Can you work these out from the model? Positions are in its coordinate system, mm. A direction names the side the tool comes from. Round coordinates to 2 decimals unless told otherwise and drop trailing zeros. Order: outer loops, then holes, each group sorted by start corner. A loop starts at its lowest first (then second) coordinate and runs counter-clockwise, first axis right, second up. Notation, with made-up numbers: (6.5, 2) - (42.5, 2) arc R16 cw to (42.5, 27) - close; hole circle Ø1 at (39.5, -34). An arc over 180 degrees is marked (long way). Write item = value, one per line.
from build123d import *

# Parameters (mm, degrees)
SKETCH1_W           = 29
SKETCH1_H           = 35
BOSS_EXTRUDE1_DEPTH = 2
SKETCH4_W           = 3
SKETCH4_H           = 35
BOSS_EXTRUDE3_DEPTH = 2
SKETCH5_W           = 3.5
SKETCH5_H           = 1.5
SKETCH5_W_2         = 1.5
SKETCH5_H_2         = 3.7
BOSS_EXTRUDE4_DEPTH = 35
SKETCH6_W           = 2
SKETCH6_H           = 35
BOSS_EXTRUDE5_DEPTH = 35
SKETCH7_W           = 32.5
SKETCH7_H           = 2
BOSS_EXTRUDE6_DEPTH = 37
CUT_EXTRUDE1_DEPTH  = 38
SKETCH11_W          = 2
SKETCH11_H          = 1.5
SKETCH11_W_2        = 3
SKETCH11_H_2        = 2
BOSS_EXTRUDE7_DEPTH = 35
SKETCH12_W          = 3.5
SKETCH12_H          = 2
SKETCH12_W_2        = 1
BOSS_EXTRUDE8_DEPTH = 35


with BuildPart() as part:
    # Sketch1 → Boss-Extrude1 (new body)
    with BuildSketch(Plane.XY):
        with Locations((0, 1.5)):
            Rectangle(SKETCH1_W, SKETCH1_H)
    extrude(amount=BOSS_EXTRUDE1_DEPTH)

    # Sketch4 → Boss-Extrude3 (add)
    with BuildSketch(Plane.XY.offset(2)):
        with Locations((-11, 1.5)):
            Rectangle(SKETCH4_W, SKETCH4_H)
        with Locations((11, 1.5)):
            Rectangle(SKETCH4_W, SKETCH4_H)
    extrude(amount=BOSS_EXTRUDE3_DEPTH)

    # Sketch5 → Boss-Extrude4 (add, through all)
    with BuildSketch(Plane(origin=(0, 19, 0), x_dir=(1, 0, 0), z_dir=(0, 1, 0))):
        Polygon((-12.5, -5.7), (-14, -5.7), (-14, -7.2), (-10.5, -7.2), (-10.5, -5.7), align=None)
        Polygon((-12.5, -4), (-12.5, -2), (-14, -2), (-14, -5.7), (-12.5, -5.7), align=None)
        with Locations((12.25, -6.45)):
            Rectangle(SKETCH5_W, SKETCH5_H)
        with Locations((13.25, -3.85)):
            Rectangle(SKETCH5_W_2, SKETCH5_H_2)
    extrude(amount=-BOSS_EXTRUDE4_DEPTH)

    # Sketch6 → Boss-Extrude5 (add)
    with BuildSketch(Plane.XY.offset(2)):
        with Locations((-13.5, 1.5)):
            Rectangle(SKETCH6_W, SKETCH6_H)
    extrude(amount=BOSS_EXTRUDE5_DEPTH)

    # Sketch7 → Boss-Extrude6 (add)
    with BuildSketch(Plane.XY):
        with Locations((1.75, -17)):
            Rectangle(SKETCH7_W, SKETCH7_H)
    extrude(amount=BOSS_EXTRUDE6_DEPTH)

    # Sketch8 → Cut-Extrude1 (cut, through all)
    with BuildSketch(Plane(origin=(0, -18, 0), x_dir=(-1, 0, 0), z_dir=(0, -1, 0))):
        with BuildLine():
            Line((6, -12), (6, -22))
            ThreePointArc((6, -22), (4.5, -23.5), (3, -22))
            Line((3, -22), (3, -12))
            ThreePointArc((3, -12), (4.5, -10.5), (6, -12))
        make_face()
    extrude(amount=-CUT_EXTRUDE1_DEPTH, mode=Mode.SUBTRACT)

    # Sketch11 → Boss-Extrude7 (add)
    with BuildSketch(Plane(origin=(0, 19, 0), x_dir=(-1, 0, 0), z_dir=(0, -1, 0))):
        with Locations((-15, -6.45)):
            Rectangle(SKETCH11_W, SKETCH11_H)
        with Locations((-15.5, -3)):
            Rectangle(SKETCH11_W_2, SKETCH11_H_2)
    extrude(amount=BOSS_EXTRUDE7_DEPTH)

    # Sketch12 → Boss-Extrude8 (add)
    with BuildSketch(Plane(origin=(0, 19, 0), x_dir=(-1, 0, 0), z_dir=(0, -1, 0))):
        with Locations((-16.25, -1)):
            Rectangle(SKETCH12_W, SKETCH12_H)
        with Locations((-17.5, -3)):
            Rectangle(SKETCH12_W_2, SKETCH12_H)
    extrude(amount=BOSS_EXTRUDE8_DEPTH)


solid = part.part
(1) Will these pins go through, and if not, where does the flat tip stop? P1, Ø6, axis at y = -1, z = 29.5, coming from the +X side; P2, Ø0.5, axis at y = 0.5, z = 5, coming from the +X side; P3, Ø2, axis at x = 1, y = 10, coming from the +Z side.
Computed:
P1 = -12.5
P2 = 14
P3 = 2
(2) If we section it at D-D (z = 33.5): Write out the boundary of the cut face in (x, y), plus the area to 3 significant figures.
Computed:
outline = (-14.5, -18) - (18, -18) - (18, -16) - (-12.5, -16) - (-12.5, 19) - (-14.5, 19) - close
area = 135 mm^2
(3) If I drill on line 1 (Z direction, x = 12, y = -3.5); line 2 (Y direction, x = 8, z = 4); line 3 (Z direction, x = -4, y = 4), over which ranges is the centre line in solid material (lowest first)? Write a range as from..to.
Computed:
line_1 = 0..4, 5.7..7.2
line_2 = -18..-16
line_3 = 0..2
(4) If we section it at C-C (y = -11): Write out the boundary of the cut face in (x, z).
Computed:
outline = (-14.5, 0) - (18, 0) - (18, 4) - (14, 4) - (14, 5.7) - (16, 5.7) - (16, 7.2) - (10.5, 7.2) - (10.5, 5.7) - (12.5, 5.7) - (12.5, 4) - (9.5, 4) - (9.5, 2) - (-9.5, 2) - (-9.5, 4) - (-12.5, 4) - (-12.5, 5.7) - (-10.5, 5.7) - (-10.5, 7.2) - (-12.5, 7.2) - (-12.5, 37) - (-14.5, 37) - close
(5) If we section it at A-A (z = 21.5): Write out the boundary of the cut face in (x, y), plus the area to 3 significant figures.
Computed:
outline = (-14.5, -18) - (-6, -18) - (-6, -16) - (-12.5, -16) - (-12.5, 19) - (-14.5, 19) - close; (-3, -18) - (18, -18) - (18, -16) - (-3, -16) - close
area = 129 mm^2
(6) Thinking about a two-plate mould opening in X: for faces 4 (the face through (-10.5, 2, 6)), 5 (the face through (2, -18, 18)), 6 (the face through (-12.5, 1, 22)), which applies, +X half, -X half, draft (parallel to the pull), parting line (faces both ways), or undercut?
Computed:
face_4 = undercut
face_5 = draft
face_6 = +X half
(7) If we section it at B-B (x = -4.5): Write out the boundary of the cut face in (y, z), plus the area to 3 significant figures.
Computed:
outline = (-18, 0) - (19, 0) - (19, 2) - (-16, 2) - (-16, 10.5) - (-18, 10.5) - close; (-18, 23.5) - (-16, 23.5) - (-16, 37) - (-18, 37) - close
area = 118 mm^2
(8) On a 3-axis mill with a long thin cutter (end or side, diameter ignored), from which of +Z, -Z, +X, -X, +Y, -Y can I reach the whole of each face in a straight line? I mean faces 1 (the face through (10.5, 2, 6)), 2 (the face through (-4.5, -17, 23.5)), 3 (the face through (11, 2, 5.7)). Say none if no direction works.
Computed:
face_1 = +Z, +Y
face_2 = +Y, -Y
face_3 = +Y
